```python
from build123d import *

# Parameters (mm, degrees)
BASPROSKE_W        = 13
BASPROSKE_H        = 17
TOOTHCUT_DEPTH     = 28.331300737
TEETHCUTS_COUNT    = 15
TEETHCUTS_ANGLE    = 336
BORSKE_R           = 4
BORE_DEPTH         = 50.0000508
SKETCH1_R          = 0.75
CUT_EXTRUDE1_DEPTH = 7
CIRPATTERN1_COUNT  = 4


with BuildPart() as part:
    # BasProSke → Base-Revolve (revolve)
    with BuildSketch(Plane(origin=(0, 0, 0), x_dir=(1, 0, 0), z_dir=(0, 1, 0)), mode=Mode.PRIVATE) as base_revolve_sk:
        with Locations((6.5, 8.5)):
            Rectangle(BASPROSKE_W, BASPROSKE_H)
    revolve(base_revolve_sk.sketch.rotate(Axis((-10, 0, 0), (1, 0, 0)), 180), axis=Axis((-10, 0, 0), (1, 0, 0)))

    # TooCutSke → ToothCut (cut, through all)
    with BuildSketch(Plane(origin=(0, 0, 0), x_dir=(0, 0, -1), z_dir=(1, 0, 0))):
        with BuildLine():
            ThreePointArc((1.050056448, 12.454813626), (0, 12.499), (-1.050056448, 12.454813626))
            ThreePointArc((-1.050056448, 12.454813626), (-1.638118106, 14.809604533), (-3.110934279, 16.73876737))
            ThreePointArc((-3.110934279, 16.73876737), (0, 17.0254), (3.110934279, 16.73876737))
            ThreePointArc((3.110934279, 16.73876737), (1.638118106, 14.809604533), (1.050056448, 12.454813626))
        make_face()
    toothcut = extrude(amount=TOOTHCUT_DEPTH, mode=Mode.SUBTRACT)

    # TeethCuts: ToothCut ×15 about axis
    teethcuts_axis = Axis((-10, 0, 0), (1, 0, 0))
    for i in range(1, TEETHCUTS_COUNT):
        add(toothcut.rotate(teethcuts_axis, i * TEETHCUTS_ANGLE / (TEETHCUTS_COUNT - 1)), mode=Mode.SUBTRACT)

    # BorSke → Bore (cut, symmetric)
    with BuildSketch(Plane(origin=(0, 0, 0), x_dir=(0, 0, -1), z_dir=(1, 0, 0))):
        with Locations(Location((0, 0, 0), (0, 0, 180))):
            Circle(BORSKE_R)
    extrude(amount=BORE_DEPTH, both=True, mode=Mode.SUBTRACT)

    # Sketch1 → Cut-Extrude1 (cut)
    with BuildSketch(Plane(origin=(13, 0, 0), x_dir=(0, 0, -1), z_dir=(1, 0, 0))):
        with Locations((-3.5, 7)):
            Circle(SKETCH1_R)
        with Locations((0, 7)):
            Circle(SKETCH1_R)
        with Locations((3.5, 7)):
            Circle(SKETCH1_R)
    cut_extrude1 = extrude(amount=-CUT_EXTRUDE1_DEPTH, mode=Mode.SUBTRACT)

    # CirPattern1: Cut-Extrude1 ×4 about axis
    cirpattern1_axis = Axis((0, 0, 0), (1, 0, 0))
    for i in range(1, CIRPATTERN1_COUNT):
        add(cut_extrude1.rotate(cirpattern1_axis, i * 360 / CIRPATTERN1_COUNT), mode=Mode.SUBTRACT)


solid = part.part
```
The listing builds one solid part. Answer for the finished solid, in the listing's coordinates (mm). A direction names the side the tool comes from. Coordinates: 2 decimals unless noted, no trailing zeros. Order: outer loops, then holes, each group sorted by start corner. A loop starts at its lowest first (then second) coordinate and runs counter-clockwise, first axis right, second up. Notation, with made-up numbers: M -2.75,47.25 L 27.25,47.25 A11 ccw 27.25,67.25 Z; hole C 39,-3 d8. An arc over 180 degrees is marked long. Answer as a JSON object with one key per item and string values. Group by question number.
1. Section D-D on x = 6.5 is taken. State how many separate pieces and enclosed holes the cut face has, then the cut area to 3 significant figures.
2. Determine the mould class of faces 5 (the cylindrical face through (6.41, -6.26, -10.82)), 6 (the cylindrical face through (6.591, 16.627, -3.541)), 7 (the cylindrical face through (6.59, 16.63, 3.53)) for opening direction Z: released by +Z, released by -Z, zero draft, split by the parting line, or undercut.
3. A tool of negligible diameter and unlimited length cuts with its end or side. For faces 1 (the cylindrical face through (6.409, -10.121, -7.335)), 2 (the flat face through (6, -7, 3)), 3 (the cylindrical face through (6.409, -14.159, 4.692)), 4 (the cylindrical face through (6.41, 12.87, -7.53)), from which of +Z, -Z, +X, -X, +Y, -Y can it reach the whole face along a straight path? Write none if from no direction.
4. Section B-B on y = 13 is taken. Write down the section's boundary in (x, z), then the cut area to 3 significant figures.
5. Section A-A on z = 0 is taken. Write down the section's boundary in (x, y).
6. Section C-C on y = 3.5 is taken. Write down the section's boundary in (x, z), then the cut area to 3 significant figures.
7. Straight lines are drawn through the part: line 1 (Z direction, x = 10.25, y = -7); line 2 (Y direction, x = 7.5, z = 0); line 3 (Y direction, x = 10.5, z = 3.5). For each, find the intervals that lie inside material, in ascending order.
8. Flat-ended cylindrical pins translate along their axes: P1, Ø6, axis at x = 2.5, z = 4.5, coming from the -Y side; P2, Ø6.5, axis at y = 0, z = 0, coming from the -X side; P3, Ø3, axis at x = 6.5, y = -12.5, coming from the -Z side. Find the tip coordinate at first contact, or state that the pin passes through.
Values follow:
{
 "1": {"separate pieces": "1", "enclosed holes": "13", "area": "602 mm2"},
 "2": {"face 5": "undercut", "face 6": "released by -Z", "face 7": "released by +Z"},
 "3": {"face 1": "+X, -X", "face 2": "+X", "face 3": "+X, -X, -Y", "face 4": "+X, -X, +Y"},
 "4": {"outline": "M 0,-10.35 L 13,-10.35 L 13,-7.69 L 0,-7.69 Z; M 0,-4.44 L 13,-4.44 L 13,-1.1 L 0,-1.1 Z; M 0,1.1 L 13,1.1 L 13,4.44 L 0,4.44 Z; M 0,7.69 L 13,7.69 L 13,10.35 L 0,10.35 Z", "area": "156 mm2"},
 "5": {"outline": "M 0,-17 L 13,-17 L 13,-7.75 L 6,-7.75 L 6,-6.25 L 13,-6.25 L 13,-4 L 0,-4 Z; M 0,4 L 13,4 L 13,6.25 L 6,6.25 L 6,7.75 L 13,7.75 L 13,12.5 L 0,12.5 Z"},
 "6": {"outline": "M 0,-12 L 13,-12 L 13,-7.75 L 6,-7.75 L 6,-6.25 L 13,-6.25 L 13,-1.94 L 0,-1.94 Z; M 0,1.94 L 13,1.94 L 13,6.25 L 6,6.25 L 6,7.75 L 13,7.75 L 13,12 L 0,12 Z", "area": "241 mm2"},
 "7": {"line 1": "-10.35 to -4.25, -2.75 to -0.75, 0.75 to 2.75, 4.25 to 10.35", "line 2": "-17 to -7.75, -6.25 to -4, 4 to 6.25, 7.75 to 12.5", "line 3": "-12 to -7.75, -6.25 to -1.94, 1.94 to 6.25, 7.75 to 16.64"},
 "8": {"P1": "y = -15.71", "P2": "through", "P3": "z = -12.93"}
}
